```python
from build123d import *

# Parameters (mm, degrees)
BOSS_EXTRUDE1_DEPTH    = 3.175
F_10_CLEARANCE_HOLE1_D = 4.9784
CUT_EXTRUDE1_DEPTH     = 160.928314508


with BuildPart() as part:
    # Sketch1 → Boss-Extrude1 (new body)
    with BuildSketch(Plane(origin=(0, 0, 0), x_dir=(0, 0, -1), z_dir=(1, 0, 0))):
        with BuildLine():
            Line((139.7, 0), (-139.7, 0))
            Line((-139.7, 0), (-139.7, 77.7875))
            Line((-139.7, 77.7875), (-127, 77.7875))
            ThreePointArc((-127, 77.7875), (-112.7125, 63.5), (-98.425, 77.7875))
            Line((-98.425, 77.7875), (-15.08125, 77.7875))
            ThreePointArc((-15.08125, 77.7875), (-0.79375, 63.5), (13.49375, 77.7875))
            Line((13.49375, 77.7875), (96.8375, 77.7875))
            ThreePointArc((96.8375, 77.7875), (111.125, 63.5), (125.4125, 77.7875))
            Line((125.4125, 77.7875), (139.7, 77.7875))
            Line((139.7, 77.7875), (139.7, 0))
        make_face()
    extrude(amount=BOSS_EXTRUDE1_DEPTH)

    # #10 Clearance Hole1 (through all)
    with Locations(Plane(origin=(3.175, 0, 0), x_dir=(0, 0, -1), z_dir=(1, 0, 0))):
        with Locations((-134.14375, 71.4375), (-91.28125, 71.4375), (-22.225, 71.4375), (20.6375, 71.4375), (89.69375, 71.4375), (132.55625, 71.4375)):
            Hole(F_10_CLEARANCE_HOLE1_D / 2)

    # Sketch4 → Cut-Extrude1 (cut, through all)
    with BuildSketch(Plane.ZY):
        with BuildLine():
            Line((-113.1189, 12.7), (-113.1189, 0))
            Line((-113.1189, 0), (-139.7, 0))
            Line((-139.7, 0), (-139.7, 38.89375))
            ThreePointArc((-139.7, 38.89375), (-135.465913951, 29.268268394), (-125.723317526, 25.31109823))
            ThreePointArc((-125.723317526, 25.31109823), (-116.810243373, 21.615031404), (-113.1189, 12.7))
        make_face()
    extrude(amount=-CUT_EXTRUDE1_DEPTH, mode=Mode.SUBTRACT)


solid = part.part
```
Read the model definition and answer for the solid it produces. Units are mm, in the model's axes. Give positions to 0.01 mm unless a question says otherwise; leave off trailing zeros. Write each loop counter-clockwise with the first axis right and the second up, starting at its lowest first coordinate (ties: lowest second). Pieces come first, ordered by that corner, then holes. Notation, with made-up numbers: (19, -9) -> (52, -9) arc R17 cw to (52, 9) -> close; hole circle Ø10 at (81, 85). An arc over 180 degrees is marked (long way). Answer as a JSON object with one key per item and string values.
1) Flat-ended cylindrical pins translate along their axes: pin 1 Ø4 at (y, z) = (71.44, 91.28) entering from +X; pin 2 Ø5.5 at (y, z) = (71.44, 134.14) entering from -X; pin 3 Ø1.6 at (x, y) = (1, 9.5) entering from -Z. Find the tip coordinate at first contact, or state that the pin passes through.
Findings below:
{"pin 1": "passes through", "pin 2": "stops at x = 0", "pin 3": "stops at z = -113.12"}
2) Section A-A on x = 0.55 is taken. Write down the section's boundary in (y, z) (1 decimal), then the cut area to 3 significant figures.
Findings below:
{"outline": "(0, -113.1) -> (12.7, -113.1) arc R12.6 cw to (25.3, -125.7) arc R14 ccw to (38.9, -139.7) -> (77.8, -139.7) -> (77.8, -125.4) arc R14.3 cw to (77.8, -96.8) -> (77.8, -13.5) arc R14.3 cw to (77.8, 15.1) -> (77.8, 98.4) arc R14.3 cw to (77.8, 127) -> (77.8, 139.7) -> (0, 139.7) -> close; hole circle Ø5 at (71.4, -132.6); hole circle Ø5 at (71.4, -89.7); hole circle Ø5 at (71.4, -20.6); hole circle Ø5 at (71.4, 22.2); hole circle Ø5 at (71.4, 91.3); hole circle Ø5 at (71.4, 134.1)", "area": "20,000 mm^2"}
3) For a pull along Y with two mould halves and no side action, classify faces 1 (the cylindrical face through (1.565, 21.713, -116.909)), 2 (the flat face through (3.175, 39, -2)), 3 (the cylindrical face through (1.57, 73.54, 23.56)), 4 (the cylindrical face through (1.565, 63.503, 113.027)) as pulls with the +Y half, pulls with the -Y half, needs draft (parallel to the pull), parting line crosses it, or undercut.
Findings below:
{"face 1": "pulls with the -Y half", "face 2": "needs draft", "face 3": "undercut", "face 4": "pulls with the +Y half"}
4) Straight lines are drawn through the part: probe 1 along Z at (x, y) = (2.2, 65.5); probe 2 along Y at (x, z) = (1.45, 1); probe 3 along Z at (x, y) = (2.9, 66). For each, find the intervals that lie inside material, in ascending order. Write a range as from..to.
Findings below:
{"probe 1": "z = -139.7..-118.42, -103.83..-6.5, 8.08..105.42, 120..139.7", "probe 2": "y = 0..63.5", "probe 3": "z = -139.7..-119.2, -103.05..-7.28, 8.87..104.64, 120.79..139.7"}
5) Section C-C on z = -8 is taken. Write down the section's boundary in (x, y) (3 decimals), then the cut area to 3 significant figures.
Findings below:
{"outline": "(0, 0) -> (3.175, 0) -> (3.175, 66.527) -> (0, 66.527) -> close", "area": "211 mm^2"}
6) Section B-B on y = 7 is taken. Write down the section's boundary in (x, z) (3 decimals), then the cut area to 3 significant figures.
Findings below:
{"outline": "(0, -113.119) -> (3.175, -113.119) -> (3.175, 139.7) -> (0, 139.7) -> close", "area": "803 mm^2"}
